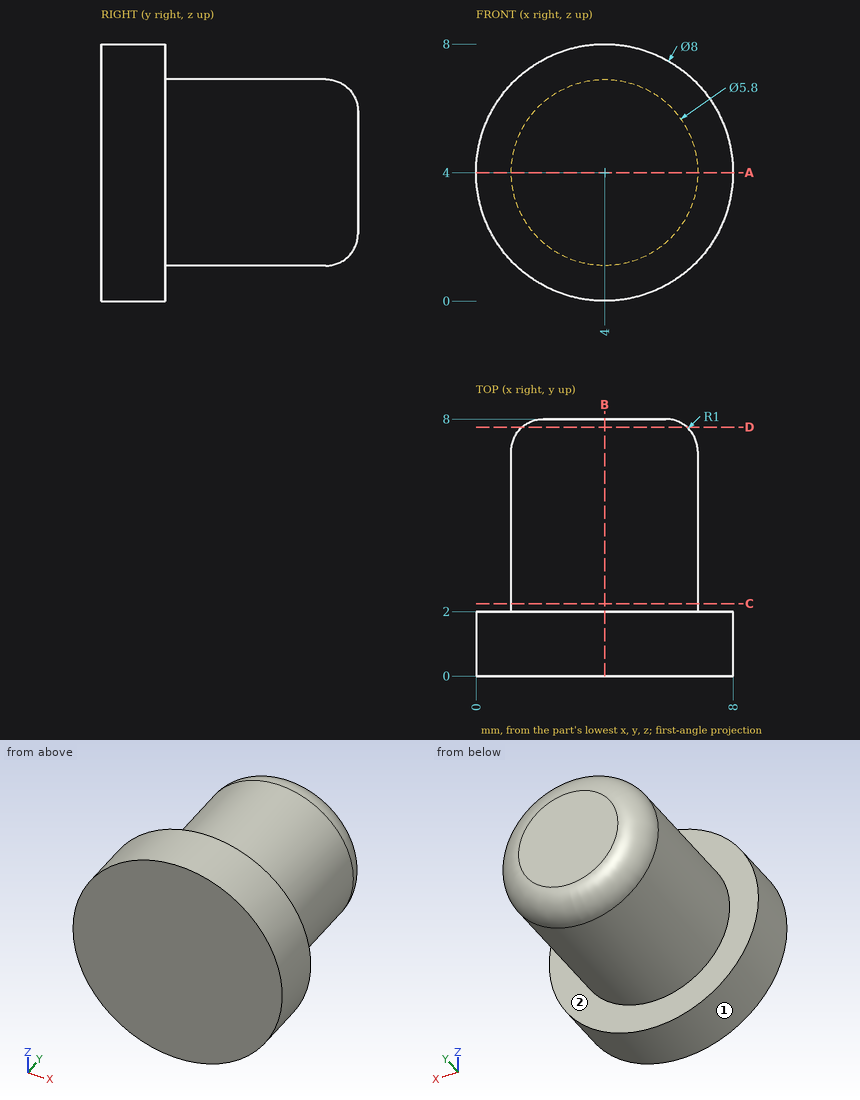
Geometry check sheet. Reference: drawing and pictorial views, mm from the part's lowest x, y, z. A direction names the side the tool comes from. Give positions to 0.01 mm unless a question says otherwise; leave off trailing zeros. Write each loop counter-clockwise with the first axis right and the second up, starting at its lowest first coordinate (ties: lowest second). Pieces come first, ordered by that corner, then holes. Notation, with made-up numbers: (73, 24) -> (111, 24) arc R11 cw to (111, 44) -> close; hole circle Ø4 at (87, 76.25). An arc over 180 degrees is marked (long way). One line per item, written item: value. Start each with the question number.
Item 1: Section check C-C on y = 2.25. Record the cut outline in (x, z), then the cut area to 3 significant figures.
Item 2: Tool access check on the marked faces 1 and 2. Record the directions out of +Z, -Z, +X, -X, +Y, -Y that give a thin tool (end or side, any length) a straight path to the whole face; none if there is none.
Item 3: Gauge pin test, flat ends, axial feed: pin 1 (2 mm diameter, centred on x = 3, z = 1, fed in from +Y) (3 decimals); pin 2 (2 mm diameter, centred on y = 2.5, z = 5, fed in from +X); pin 3 (1.5 mm diameter, centred on x = 1, z = 3, fed in from +Y). Record the tip position at first contact, or that the pin passes through.
Item 4: Material ranges on probe 1 along Y at (x, z) = (1.25, 6.75); probe 2 along Z at (x, y) = (5, 0.5); probe 3 along X at (y, z) = (1, 2.25), recorded low to high. Write a range as from..to.
Item 5: Section check D-D on y = 7.75. Record the cut outline in (x, z).
Item 6: Section check B-B on x = 4. Record the cut outline in (y, z).
Item 7: Section check A-A on z = 4. Record the cut outline in (x, y).
Results list:
1. outline: circle Ø5.8 at (4, 4)
1. area: 26.4 mm²
2. face 1: +Y, -Y
2. face 2: +Y
3. pin 1: y = 7.965
3. pin 2: x = 8
3. pin 3: y = 7.86
4. probe 1: 0..2
4. probe 2: 0.13..7.87
4. probe 3: 0.4..7.6
5. outline: circle Ø5.12 at (4, 4)
6. outline: (0, 0) -> (2, 0) -> (2, 1.1) -> (7, 1.1) arc R1 ccw to (8, 2.1) -> (8, 5.9) arc R1 ccw to (7, 6.9) -> (2, 6.9) -> (2, 8) -> (0, 8) -> close
7. outline: (0, 0) -> (8, 0) -> (8, 2) -> (6.9, 2) -> (6.9, 7) arc R1 ccw to (5.9, 8) -> (2.1, 8) arc R1 ccw to (1.1, 7) -> (1.1, 2) -> (0, 2) -> close
